Here's how the part is built. I have some questions about the finished solid (model axes, mm). Round coordinates to 2 decimals unless told otherwise and drop trailing zeros. Write each loop counter-clockwise with the first axis right and the second up, starting at its lowest first coordinate (ties: lowest second). Pieces come first, ordered by that corner, then holes. Notation, with made-up numbers: (51.5, 10) -> (61.5, 10) arc R17 cw to (61.5, 29) -> close; hole circle Ø4 at (-16.5, 60.25). An arc over 180 degrees is marked (long way). Put each result on its own line as item: value. Start each with the question number.
1) I want a section at D-D, the plane y = -34. List the corners of the cut face in (x, z) for me.
2) Will this pin go through, and if not, where does the flat tip stop? P1, Ø10, axis at x = -15, y = -10, coming from the -Z side.
3) I want a section at B-B, the plane y = -75. List the corners of the cut face in (x, z) for me, then the cut area to 3 significant figures.
4) I want a section at A-A, the plane x = 36. List the corners of the cut face in (y, z) for me, then the cut area to 3 significant figures.
5) If I drill on line 1 along X through (y, z) = (-26, 2); line 2 along Y through (x, z) = (36, 1.9); line 3 along X through (y, z) = (3.5, 1.55), over which ranges is the centre line in solid material (lowest first)? Write a range as [from, to].
6) I want a section at C-C, the plane z = 1.85. List the corners of the cut face in (x, y) for me, then the cut area to 3 significant figures.
from build123d import *

# Parameters (mm, degrees)
SKETCH1_W           = 150
SKETCH1_H           = 160
BOSS_EXTRUDE1_DEPTH = 3.2
CUT_EXTRUDE1_REACH  = 5.2
CUT_EXTRUDE2_REACH  = 5.2
SKETCH3_R           = 2.75


with BuildPart() as part:
    # Sketch1 → Boss-Extrude1 (new body)
    with BuildSketch(Plane.XY):
        Rectangle(SKETCH1_W, SKETCH1_H)
    extrude(amount=BOSS_EXTRUDE1_DEPTH)

    # Sketch2 → Cut-Extrude1 (cut, up to next)
    with BuildSketch(Plane.XY.offset(3.2), mode=Mode.PRIVATE) as cut_extrude1_sk1:
        with BuildLine():
            Line((-25, -12), (-25, -80))
            Line((-25, -80), (25, -80))
            Line((25, -80), (25, -12))
            ThreePointArc((25, -12), (0, 13), (-25, -12))
        make_face()
    cut_extrude1_tool1 = extrude(cut_extrude1_sk1.sketch, amount=-CUT_EXTRUDE1_REACH, mode=Mode.PRIVATE) & part.part
    add(cut_extrude1_tool1.solids().sort_by_distance((0, -36.004881, 3.2))[0], mode=Mode.SUBTRACT)

    # Sketch3 → Cut-Extrude2 (cut, up to next)
    with BuildSketch(Plane.XY.offset(3.2), mode=Mode.PRIVATE) as cut_extrude2_sk1:
        with Locations((36, -75)):
            Circle(SKETCH3_R)
    cut_extrude2_tool1 = extrude(cut_extrude2_sk1.sketch, amount=-CUT_EXTRUDE2_REACH, mode=Mode.PRIVATE) & part.part
    add(cut_extrude2_tool1.solids().sort_by_distance((36, -75, 3.2))[0], mode=Mode.SUBTRACT)
    # Sketch3 → Cut-Extrude2 (cut, up to next)
    with BuildSketch(Plane.XY.offset(3.2), mode=Mode.PRIVATE) as cut_extrude2_sk2:
        with Locations((-36, -75)):
            Circle(SKETCH3_R)
    cut_extrude2_tool2 = extrude(cut_extrude2_sk2.sketch, amount=-CUT_EXTRUDE2_REACH, mode=Mode.PRIVATE) & part.part
    add(cut_extrude2_tool2.solids().sort_by_distance((-36, -75, 3.2))[0], mode=Mode.SUBTRACT)
    # Sketch3 → Cut-Extrude2 (cut, up to next)
    with BuildSketch(Plane.XY.offset(3.2), mode=Mode.PRIVATE) as cut_extrude2_sk3:
        Polygon((-41, 20), (-41, -80), (-75, -80), (-75, 80), (75, 80), (75, -80), (41, -80), (41, 20), align=None)
    cut_extrude2_tool3 = extrude(cut_extrude2_sk3.sketch, amount=-CUT_EXTRUDE2_REACH, mode=Mode.PRIVATE) & part.part
    add(cut_extrude2_tool3.solids().sort_by_distance((-43.193171, -30, 3.2))[0], mode=Mode.SUBTRACT)


solid = part.part
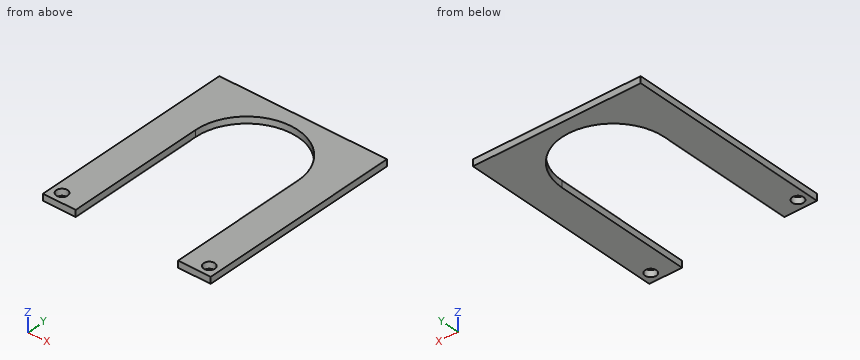
Findings:
1. outline: (-41, 0) -> (-25, 0) -> (-25, 3.2) -> (-41, 3.2) -> close; (25, 0) -> (41, 0) -> (41, 3.2) -> (25, 3.2) -> close
2. P1: passes through
3. outline: (-41, 0) -> (-38.75, 0) -> (-38.75, 3.2) -> (-41, 3.2) -> close; (-33.25, 0) -> (-25, 0) -> (-25, 3.2) -> (-33.25, 3.2) -> close; (25, 0) -> (33.25, 0) -> (33.25, 3.2) -> (25, 3.2) -> close; (38.75, 0) -> (41, 0) -> (41, 3.2) -> (38.75, 3.2) -> close
3. area: 67.2 mm2
4. outline: (-80, 0) -> (-77.75, 0) -> (-77.75, 3.2) -> (-80, 3.2) -> close; (-72.25, 0) -> (20, 0) -> (20, 3.2) -> (-72.25, 3.2) -> close
4. area: 302 mm2
5. line 1: x = [-41, -25], [25, 41]
5. line 2: y = [-80, -77.75], [-72.25, 20]
5. line 3: x = [-41, -19.62], [19.62, 41]
6. outline: (-41, -80) -> (-25, -80) -> (-25, -12) arc R25 cw to (25, -12) -> (25, -80) -> (41, -80) -> (41, 20) -> (-41, 20) -> close; hole circle Ø5.5 at (-36, -75); hole circle Ø5.5 at (36, -75)
6. area: 3,770 mm2
